For this review, take the finished solid that the model builds, in its own axes (mm). Face numbers are marked on the shaded views. A direction names the side the tool comes from. Round coordinates to 2 decimals unless told otherwise and drop trailing zeros. Write each loop counter-clockwise with the first axis right and the second up, starting at its lowest first coordinate (ties: lowest second). Pieces come first, ordered by that corner, then holes. Notation, with made-up numbers: (43, 23) -> (54, 23) arc R13 ccw to (54, 33) -> close; hole circle Ø10 at (-20.5, 41). An arc over 180 degrees is marked (long way). Answer as CSV lines item,"result". Start each with the question number.
Item 1: Wall thickness on probe 1 along Y at (x, z) = (-26.5, -11.5); probe 2 along X at (y, z) = (11, -19.75); probe 3 along Y at (x, z) = (0, -20.9): over which ranges is each line inside the solid? List them lowest first. Write a range as from..to.
Item 2: Take a section at B-B on x = 18. Give the boundary of the cut face in (y, z), then the cut area to 3 significant figures.
Item 3: Take a section at A-A on y = 0. Give the boundary of the cut face in (x, z).
Item 4: Machinability: for the marked faces 1, 2 and 3, which of the approach directions +Z, -Z, +X, -X, +Y, -Y give a long, thin tool a straight path to every point of the face, cutting with its end or side? Answer none if there is none.
Item 5: Take a section at C-C on y = 37. Give the boundary of the cut face in (x, z), then the cut area to 3 significant figures.
Item 6: Mouldability with a two-part tool opening along X and no side actions: class the marked faces 4, 5 and 6 as +X half, -X half, draft (parallel to the pull), parting line (faces both ways), or undercut.
Item 7: Take a section at D-D on z = -12.75. Give the boundary of the cut face in (x, y).
Item 8: For pin 1 Ø2.5 at (x, y) = (10.5, -1) entering from +Z; pin 2 Ø8 at (y, z) = (20, -16) entering from -X; pin 3 Ø3 at (y, z) = (-1, -19) entering from +X, all flat-tipped, find the tip position at first contact; note any pin that passes through.
```python
from build123d import *

# Parameters (mm, degrees)
F0_W      = 58.5
F0_H      = 91
F1_DEPTH  = 22
F2_T      = -1.5
F3_R      = 3
F4_R      = 2
F5_R      = 4
F6_DEPTH  = 22
F7_R      = 1.8
F8_DEPTH  = 20
F11_W     = 28
F11_H     = 10
F11_W_2   = 24
F11_H_2   = 6
F12_DEPTH = 4
F10_R     = 10.25
F13_DEPTH = 25


with BuildPart() as f1:
    # F0 (on Top) → F1 (new body)
    with BuildSketch(Plane.XY):
        Rectangle(F0_W, F0_H)
    extrude(amount=-F1_DEPTH)

    # F2
    f2_openings = [f1.faces().sort_by_distance(p)[0] for p in [
        (0, 0, 0),
    ]]
    offset(amount=F2_T, openings=f2_openings)

    # F3
    f3_edges = [f1.edges().sort_by_distance(p)[0] for p in [
        (-29.25, 45.5, -11),
        (29.25, 45.5, -11),
        (-29.25, -45.5, -11),
        (29.25, -45.5, -11),
    ]]
    fillet(f3_edges, radius=F3_R)

    # F4
    f4_edges = [f1.edges().sort_by_distance(p)[0] for p in [
        (-27.75, 44, -10.25),
        (-27.75, -44, -10.25),
        (27.75, -44, -10.25),
        (27.75, 44, -10.25),
    ]]
    fillet(f4_edges, radius=F4_R)

    # F5 (on face) → F6 (join)
    with BuildSketch(Plane.XY):
        with Locations((26.5, -42.5)):
            Circle(F5_R)
        with Locations((26.5, 42.5)):
            Circle(F5_R)
        with Locations((-26.5, 42.5)):
            Circle(F5_R)
        with Locations((-26.5, -42.5)):
            Circle(F5_R)
    extrude(amount=-F6_DEPTH)

    # F7 (on Top) → F8 (cut)
    with BuildSketch(Plane.XY):
        with Locations((26.5, -42.5)):
            Circle(F7_R)
        with Locations((26.5, 42.5)):
            Circle(F7_R)
        with Locations((-26.5, -42.5)):
            Circle(F7_R)
        with Locations((-26.5, 42.5)):
            Circle(F7_R)
    extrude(amount=-F8_DEPTH, mode=Mode.SUBTRACT)

    # F11 (on face) → F12 (join)
    with BuildSketch(Plane(origin=(0, 0, -22), x_dir=(1, 0, 0), z_dir=(0, 0, -1))):
        Rectangle(F11_W, F11_H)
        Rectangle(F11_W_2, F11_H_2, mode=Mode.SUBTRACT)
    extrude(amount=-F12_DEPTH)

    # F10 (on face) → F13 (cut)
    with BuildSketch(Plane(origin=(0, 0, -22), x_dir=(1, 0, 0), z_dir=(0, 0, -1))):
        Circle(F10_R)
    extrude(amount=-F13_DEPTH, mode=Mode.SUBTRACT)


solid = f1.part
```
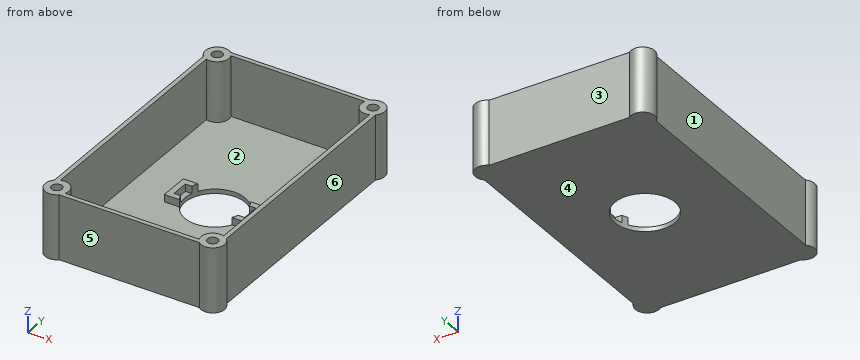
Output values:
1,probe 1,"y = -46.5..-44.3, -40.7..-38.5, 38.5..40.7, 44.3..46.5"
1,probe 2,"x = -29.25..-27.75, 27.75..29.25"
1,probe 3,"y = -45.5..-10.25, 10.25..45.5"
2,outline,"(-45.5, -22) -> (45.5, -22) -> (45.5, 0) -> (44, 0) -> (44, -20.5) -> (-44, -20.5) -> (-44, 0) -> (-45.5, 0) -> close"
2,area,"198 mm^2"
3,outline,"(-29.25, -22) -> (-10.25, -22) -> (-10.25, -20.5) -> (-12, -20.5) -> (-12, -18) -> (-14, -18) -> (-14, -20.5) -> (-27.75, -20.5) -> (-27.75, 0) -> (-29.25, 0) -> close; (10.25, -22) -> (29.25, -22) -> (29.25, 0) -> (27.75, 0) -> (27.75, -20.5) -> (14, -20.5) -> (14, -18) -> (12, -18) -> (12, -20.5) -> (10.25, -20.5) -> close"
4,face 1,"+Z, -Z, -X"
4,face 2,"+Z"
4,face 3,"+Z, -Z, +Y"
5,outline,"(-29.25, -22) -> (29.25, -22) -> (29.25, 0) -> (27.75, 0) -> (27.75, -20.5) -> (-27.75, -20.5) -> (-27.75, 0) -> (-29.25, 0) -> close"
5,area,"149 mm^2"
6,face 4,"draft"
6,face 5,"undercut"
6,face 6,"+X half"
7,outline,"(-29.25, -39.6) arc R4 ccw to (-23.85, -45.5) -> (23.85, -45.5) arc R4 ccw to (29.25, -39.6) -> (29.25, 39.6) arc R4 ccw to (23.85, 45.5) -> (-23.85, 45.5) arc R4 ccw to (-29.25, 39.6) -> close; hole circle Ø3.6 at (-26.5, -42.5); hole circle Ø3.6 at (-26.5, 42.5); hole (-27.75, -38.7) arc R4 cw to (-22.79, -44) -> (22.79, -44) arc R4 cw to (27.75, -38.7) -> (27.75, 38.7) arc R4 cw to (22.79, 44) -> (-22.79, 44) arc R4 cw to (-27.75, 38.7) -> close; hole circle Ø3.6 at (26.5, -42.5); hole circle Ø3.6 at (26.5, 42.5)"
8,pin 1,"stops at z = -20.5"
8,pin 2,"stops at x = -29.25"
8,pin 3,"stops at x = 29.25"
